from build123d import *

# Parameters (mm, degrees)
SKETCH1_R           = 5
BOSS_EXTRUDE1_DEPTH = 200
SKETCH2_R           = 2.5
CUT_EXTRUDE1_DEPTH  = 6


with BuildPart() as part:
    # Sketch1 → Boss-Extrude1 (new body)
    with BuildSketch(Plane.XY):
        Polygon((-12.5, 11.990821063), (-12.5, -12.5), (12.5, -12.5), (12.5, 5.5), (2.5, 5.5), (2.5, 11), (2.498974596, 11.001776051), (1.633974596, 12.5), (0.768974596, 11.001776051), (-0.096025404, 12.5), (-0.961025404, 11.001776051), (-1.826025404, 12.5), (-2.691025404, 11.001776051), (-3.556025404, 12.5), (-4.421025404, 11.001776051), (-5.286025404, 12.5), (-6.151025404, 11.001776051), (-7.016025404, 12.5), (-7.881025404, 11.001776051), (-8.746025404, 12.5), (-9.611025404, 11.001776051), (-10.476025404, 12.5), (-11.341025404, 11.001776051), (-12.206025404, 12.5), align=None)
        with Locations((-5, 0)):
            Circle(SKETCH1_R, mode=Mode.SUBTRACT)
    extrude(amount=BOSS_EXTRUDE1_DEPTH)

    # Sketch2 → Cut-Extrude1 (cut)
    with BuildSketch(Plane.XZ.offset(12.5)):
        with Locations(Location((0, 140, 0), (0, 0, 270))):
            Circle(SKETCH2_R)
        with Locations(Location((0, 60, 0), (0, 0, 90))):
            Circle(SKETCH2_R)
    extrude(amount=-CUT_EXTRUDE1_DEPTH, mode=Mode.SUBTRACT)


solid = part.part
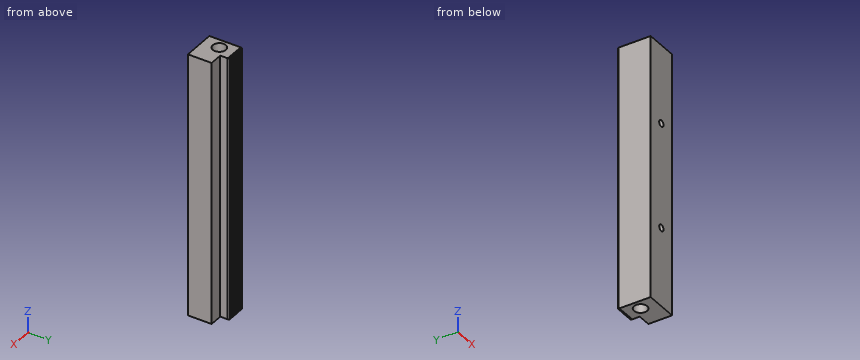
Could you check a few things on this model? Use its own coordinates, in mm. Coordinates: 2 decimals unless noted, no trailing zeros. Write each loop counter-clockwise with the first axis right and the second up, starting at its lowest first coordinate (ties: lowest second). Pieces come first, ordered by that corner, then holes. Notation, with made-up numbers: M -28,3 L 11,3 A19 cw 11,39 Z; hole C -33.75,48 d4. An arc over 180 degrees is marked long. One line per question, with ' | ' between items.
1) For pin 1 Ø6 at (x, z) = (0, 60) entering from -Y; pin 2 Ø2.5 at (x, z) = (0.5, 59.5) entering from -Y; pin 3 Ø8 at (x, z) = (5.5, 69) entering from +Y; pin 4 Ø1.6 at (y, z) = (8.5, 109.5) entering from +X, each with a flat end and sliding along its axis, tell me the tip position at first contact or that it passes through.
Checks:
pin 1: y = -12.5 | pin 2: y = -6.5 | pin 3: y = 12.5 | pin 4: x = 2.5
2) Imagine slicing it at C-C, the plane x = 9.75. Write out the boundary of the cut face in (y, z).
Checks:
outline: M -12.5,0 L 5.5,0 L 5.5,200 L -12.5,200 Z
3) Imagine slicing it at A-A, the plane y = 0. Write out the boundary of the cut face in (x, z).
Checks:
outline: M -12.5,0 L -10,0 L -10,200 L -12.5,200 Z; M 0,0 L 12.5,0 L 12.5,200 L 0,200 Z
4) I need wall thicknesses on probe 1 along X at (y, z) = (-8.4, 140); probe 2 along Y at (x, z) = (-5, 61); probe 3 along X at (y, z) = (10.25, 140). Which ranges of each line are inside material? Lowest first, please. Write a range as [from, to].
Checks:
probe 1: [-12.5, -2.5], [2.5, 12.5] | probe 2: [-12.5, -5], [5, 12] | probe 3: [-12.5, 2.5]
